from build123d import *

# Parameters (mm, degrees)
SKETCH_R        = 40
SKETCH_R_2      = 10.5
PAD_DEPTH       = 30
SKETCH001_R     = 5
POCKET_DEPTH    = 75.804681
SKETCH002_W     = 60
SKETCH002_H     = 20
POCKET001_DEPTH = 10
SKETCH003_R     = 40
SKETCH003_R_2   = 30
PAD001_DEPTH    = 60


with BuildPart() as part:
    # Sketch → Pad (new body)
    with BuildSketch(Plane.XZ):
        with BuildLine():
            ThreePointArc((-29.333333, -46.524784), (0, -55), (29.333333, -46.524784))
            Line((29.333333, -46.524784), (72.266667, -19.455819))
            ThreePointArc((72.266667, -19.455819), (82.97229, -1.128676), (74.114792, 18.159644))
            Line((74.114792, 18.159644), (42.726268, 42.556734))
            ThreePointArc((35, 58.347728), (37.035109, 49.557809), (42.726268, 42.556734))
            Line((35, 75.803681), (35, 58.347728))
            Line((-35, 75.803681), (35, 75.803681))
            Line((-35, 58.347728), (-35, 75.803681))
            ThreePointArc((-42.726268, 42.556734), (-37.035109, 49.557809), (-35, 58.347728))
            Line((-74.114792, 18.159644), (-42.726268, 42.556734))
            ThreePointArc((-74.114792, 18.159644), (-82.97229, -1.128676), (-72.266667, -19.455819))
            Line((-72.266667, -19.455819), (-29.333333, -46.524784))
        make_face()
        Circle(SKETCH_R, mode=Mode.SUBTRACT)
        with Locations((-60, 0)):
            Circle(SKETCH_R_2, mode=Mode.SUBTRACT)
        with Locations((60, 0)):
            Circle(SKETCH_R_2, mode=Mode.SUBTRACT)
    extrude(amount=-PAD_DEPTH)

    # Sketch001 → Pocket (cut, through all)
    with BuildSketch(Plane.XY):
        with Locations((0, 15)):
            Circle(SKETCH001_R)
    extrude(amount=POCKET_DEPTH, mode=Mode.SUBTRACT)

    # Sketch002 (on Face13 of Pocket) → Pocket001 (cut)
    with BuildSketch(Plane(origin=(0, 0, 75.803681), x_dir=(-1, 0, 0), z_dir=(0, 0, 1))):
        with Locations((0, -15)):
            Rectangle(SKETCH002_W, SKETCH002_H)
    extrude(amount=-POCKET001_DEPTH, mode=Mode.SUBTRACT)

    # Sketch003 (on DatumPlane) → Pad001 (join)
    with BuildSketch(Plane.XZ.offset(5)):
        Circle(SKETCH003_R)
        Circle(SKETCH003_R_2, mode=Mode.SUBTRACT)
    extrude(amount=-PAD001_DEPTH)


solid = part.part
Can you work these out from the model? Positions are in its coordinate system, mm. A direction names the side the tool comes from. Coordinates: 2 decimals unless noted, no trailing zeros. Loops run counter-clockwise (first coordinate to the right, second up) from the corner with the lowest first, then second, coordinate; pieces in that order, holes last. Notation, with made-up numbers: M 74.25,70.5 L 129.25,70.5 A32 cw 129.25,97.5 Z; hole C 19.25,24.25 d11. An arc over 180 degrees is marked long. Return JSON: item names as keys, results as strings. Group by question number.
Item 1: Imagine slicing it at B-B (y = 15). Please give me the cut outline in (x, z), and give its area (3 significant figures).
Item 2: Imagine slicing it at A-A (x = 0). Please give me the cut outline in (y, z).
Item 3: If I drill on L1, parallel to X at y = 15, z = 59; L2, parallel to X at y = 20, z = -7.5; L3, parallel to Y at x = 0, z = 59.5, over which ranges is the centre line in solid material (lowest first)? Write a range as from..to.
Item 4: I'm going to push flat-ended pins straight in: pin 1 Ø1 at (y, z) = (5, 37.5) entering from +X; pin 2 Ø8 at (x, z) = (22.5, -4) entering from -Y; pin 3 Ø3 at (x, z) = (9, 71.5) entering from -Y; pin 4 Ø1 at (y, z) = (42, -8) entering from +X. Where does each tip first touch, or does it pass through?
Item 5: Imagine slicing it at D-D (y = 32.5). Please give me the cut outline in (x, z), and give its area (3 significant figures).
Item 6: On a 3-axis mill with a long thin cutter (end or side, diameter ignored), from which of +Z, -Z, +X, -X, +Y, -Y can I reach the whole of each face in a straight line? I mean faces 5 (the flat face through (-30, 15, 71)), 6 (the cylindrical face through (82.955, 14.79, -1.437)), 7 (the flat face through (-1.2, 0, 40.4)). Say none if no direction works.
Item 7: Thinking about a two-plate mould opening in Y: for faces 1 (the flat face through (7, 15, 65.804)), 2 (the cylindrical face through (-82.985, 14.79, -0.82)), 3 (the cylindrical face through (-1.08, 10.12, 52.56)), 4 (the flat face through (6, 55, 30)), which applies, released by +Y, released by -Y, zero draft, split by the parting line, or undercut?
Item 8: Imagine slicing it at C-C (z = -6). Please give me the cut outline in (x, y), and give its area (3 significant figures).
Verdict:
{
 "1": {"outline": "M -74.11,18.16 A23 ccw -72.27,-19.46 L -29.33,-46.52 A55 ccw 29.33,-46.52 L 72.27,-19.46 A23 ccw 74.11,18.16 L 42.73,42.56 A20 cw 35,58.35 L 35,75.8 L 30,75.8 L 30,65.8 L 5,65.8 L 5,39.69 A40 ccw -5,39.69 L -5,65.8 L -30,65.8 L -30,75.8 L -35,75.8 L -35,58.35 A20 cw -42.73,42.56 Z; hole C -60,0 d21; hole C 0,0 d60; hole C 60,0 d21", "area": "9,980 mm^2"},
 "2": {"outline": "M -5,-40 L 0,-40 L 0,-55 L 30,-55 L 30,-40 L 55,-40 L 55,-30 L -5,-30 Z; M -5,30 L 55,30 L 55,40 L 30,40 L 30,75.8 L 25,75.8 L 25,65.8 L 20,65.8 L 20,40 L 10,40 L 10,65.8 L 5,65.8 L 5,75.8 L 0,75.8 L 0,40 L -5,40 Z"},
 "3": {"L1": "x = -35..-5, 5..35", "L2": "x = -81.74..-67.35, -52.65..-29.05, 29.05..52.65, 67.35..81.74", "L3": "y = 0..10, 20..30"},
 "4": {"pin 1": "stops at x = 49.88", "pin 2": "passes through", "pin 3": "stops at y = 0", "pin 4": "stops at x = 39.29"},
 "5": {"outline": "C 0,0 d80; hole C 0,0 d60", "area": "2,200 mm^2"},
 "6": {"face 5": "+Z", "face 6": "+X, +Y, -Y", "face 7": "-Y"},
 "7": {"face 1": "undercut", "face 2": "zero draft", "face 3": "undercut", "face 4": "released by +Y"},
 "8": {"outline": "M -82.2,0 L -68.62,0 L -68.62,30 L -82.2,30 Z; M -51.38,0 L -39.55,0 L -39.55,-5 L -29.39,-5 L -29.39,55 L -39.55,55 L -39.55,30 L -51.38,30 Z; M 29.39,-5 L 39.55,-5 L 39.55,0 L 51.38,0 L 51.38,30 L 39.55,30 L 39.55,55 L 29.39,55 Z; M 68.62,0 L 82.2,0 L 82.2,30 L 68.62,30 Z", "area": "2,740 mm^2"}
}
